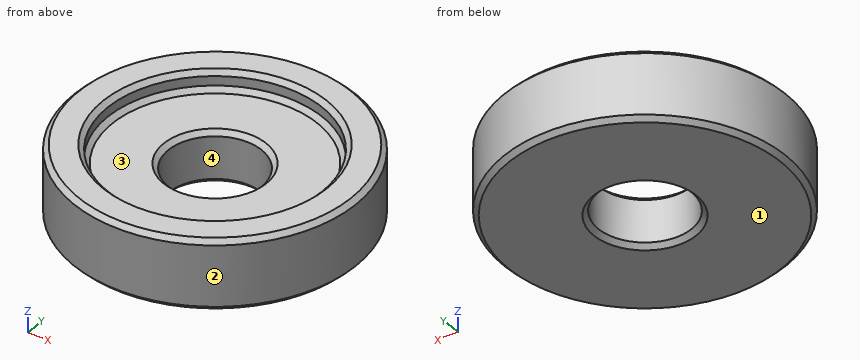
from build123d import *

# Parameters (mm, degrees)
SKETCH2_R           = 15.1
SKETCH2_R_2         = 5
BOSS_EXTRUDE1_DEPTH = 7.5
SKETCH3_R           = 11.5
CUT_EXTRUDE1_DEPTH  = 2
CHAMFER1_SIZE       = 0.5


with BuildPart() as part:
    # Sketch2 → Boss-Extrude1 (new body)
    with BuildSketch(Plane.XY):
        Circle(SKETCH2_R)
        Circle(SKETCH2_R_2, mode=Mode.SUBTRACT)
    extrude(amount=BOSS_EXTRUDE1_DEPTH)

    # Sketch3 → Cut-Extrude1 (cut)
    with BuildSketch(Plane.XY.offset(7.5)):
        Circle(SKETCH3_R)
    extrude(amount=-CUT_EXTRUDE1_DEPTH, mode=Mode.SUBTRACT)

    # Chamfer1
    chamfer1_edges = [part.edges().sort_by_distance(p)[0] for p in [
        (-11.5, 0, 5.5),
        (-5, 0, 5.5),
        (-11.5, 0, 7.5),
        (-15.1, 0, 0),
        (-15.1, 0, 7.5),
        (-5, 0, 0),
    ]]
    chamfer(chamfer1_edges, length=CHAMFER1_SIZE)


solid = part.part
The listing builds one solid part. Answer for the finished solid, in the listing's coordinates (mm). Face numbers are marked on the shaded views. Coordinates: 2 decimals unless noted, no trailing zeros. Loops run counter-clockwise (first coordinate to the right, second up) from the corner with the lowest first, then second, coordinate; pieces in that order, holes last.
1) Determine the mould class of the marked faces 1, 2, 3 and 4 for opening direction Y: pulls with the +Y half, pulls with the -Y half, needs draft (parallel to the pull), parting line crosses it, or undercut.
2) Flat-ended cylindrical pins translate along their axes: pin 1 Ø3 at (y, z) = (-5, 2.5) entering from -X; pin 2 Ø9 at (x, y) = (0, 0) entering from -Z; pin 3 Ø4 at (x, y) = (-4.5, 8) entering from +Z; pin 4 Ø8 at (x, y) = (4, 4) entering from +Z. Find the tip coordinate at first contact, or state that the pin passes through.
3) Find the intervals of material crossed by L1, parallel to Y at x = 0, z = 2.25; L2, parallel to Y at x = 0, z = 6.35; L3, parallel to Z at x = -3.5, y = 10, in increasing order.
4) Find section A-A on x = 0. Write down the section's boundary in (y, z).
5) Find section C-C on z = 2.25. Write down the section's boundary in (x, y).
Values:
1. face 1: needs draft
1. face 2: parting line crosses it
1. face 3: undercut
1. face 4: undercut
2. pin 1: stops at x = -14.69
2. pin 2: passes through
2. pin 3: stops at z = 5.68
2. pin 4: stops at z = 5.5
3. L1: y = -15.1 to -5, 5 to 15.1
3. L2: y = -15.1 to -11.5, 11.5 to 15.1
3. L3: z = 0 to 5.5
4. outline: (-15.1, 0.5) - (-14.6, 0) - (-5.5, 0) - (-5, 0.5) - (-5, 5) - (-5.5, 5.5) - (-11, 5.5) - (-11.5, 6) - (-11.5, 7) - (-12, 7.5) - (-14.6, 7.5) - (-15.1, 7) - close; (5, 0.5) - (5.5, 0) - (14.6, 0) - (15.1, 0.5) - (15.1, 7) - (14.6, 7.5) - (12, 7.5) - (11.5, 7) - (11.5, 6) - (11, 5.5) - (5.5, 5.5) - (5, 5) - close
5. outline: circle Ø30.2 at (0, 0); hole circle Ø10 at (0, 0)
